Geometry: final body of the model. Coordinates: model frame, mm. Give positions to 0.01 mm unless a question says otherwise; leave off trailing zeros. Order: outer loops, then holes, each group sorted by start corner. A loop starts at its lowest first (then second) coordinate and runs counter-clockwise, first axis right, second up. Notation, with made-up numbers: M 87,-25.5 L 123,-25.5 A18 ccw 123,-17.5 Z; hole C 59,77.25 d11. An arc over 180 degrees is marked long. Write item = value, one per line. Start each with the question number.
from build123d import *

# Parameters (mm, degrees)
SKETCH2_W            = 13.3
SKETCH2_H            = 12
SKETCH2_W_2          = 40.4
BOSS_EXTRUDE1_DEPTH  = 8.000000075
M3_CLEARANCE_HOLE1_D = 3.6


with BuildPart() as part:
    # Sketch2 → Boss-Extrude1 (new body)
    with BuildSketch(Plane.XY):
        with Locations((74.00000003, 44.5)):
            Rectangle(SKETCH2_W, SKETCH2_H)
        with Locations((100.85000003, 44.5)):
            Rectangle(SKETCH2_W_2, SKETCH2_H)
        with Locations((127.70000003, 44.5)):
            Rectangle(SKETCH2_W, SKETCH2_H)
    extrude(amount=BOSS_EXTRUDE1_DEPTH)

    # M3 Clearance Hole1 (through all)
    with Locations(Plane(origin=(2.6e-08, 0, 8.00000029), x_dir=(1.0, 0, -3.199998676446638e-09), z_dir=(3.199998676446638e-09, 0, 1.0))):
        with Locations((70.750000016, 47), (130.750000016, 47)):
            Hole(M3_CLEARANCE_HOLE1_D / 2)


solid = part.part
1) Cut plane A-A (x = 130.75). Return loops of the section in (y, z).
2) Draft query along Y for faces 1 (the flat face through (100, 38.5, 4)), 2 (the cylindrical face through (129.782, 48.518, 3.944)), 3 (the flat face through (100, 45, 0)). Return one class per face: pulls with the +Y half, pulls with the -Y half, needs draft (parallel to the pull), parting line crosses it, or undercut.
3) Ray query, L1, parallel to Y at x = 70.75, z = 4.25; L2, parallel to X at y = 48, z = 3.5; L3, parallel to X at y = 45.75, z = 2.25. Return the intervals inside material, ascending.
4) Cut plane C-C (z = 3). Return loops of the section in (x, y).
5) Cut plane B-B (y = 47). Return loops of the section in (x, z), plus the area to 3 significant figures.
Reply:
q1.outline = M 38.5,0 L 45.2,0 L 45.2,8 L 38.5,8 Z; M 48.8,0 L 50.5,0 L 50.5,8 L 48.8,8 Z
q2.face_1 = pulls with the -Y half
q2.face_2 = undercut
q2.face_3 = needs draft
q3.L1 = 38.5 to 45.2, 48.8 to 50.5
q3.L2 = 67.35 to 69.25, 72.25 to 129.25, 132.25 to 134.35
q3.L3 = 67.35 to 69.45, 72.05 to 129.45, 132.05 to 134.35
q4.outline = M 67.35,38.5 L 134.35,38.5 L 134.35,50.5 L 67.35,50.5 Z; hole C 70.75,47 d3.6; hole C 130.75,47 d3.6
q5.outline = M 67.35,0 L 68.95,0 L 68.95,8 L 67.35,8 Z; M 72.55,0 L 128.95,0 L 128.95,8 L 72.55,8 Z; M 132.55,0 L 134.35,0 L 134.35,8 L 132.55,8 Z
q5.area = 478 mm²
